Geometry: final body of the model. Coordinates: model frame, mm. Face numbers are marked on the shaded views. A direction names the side the tool comes from. Coordinates: 2 decimals unless noted, no trailing zeros. Loops run counter-clockwise (first coordinate to the right, second up) from the corner with the lowest first, then second, coordinate; pieces in that order, holes last. Notation, with made-up numbers: (-17.5, -11.5) - (-13.5, -11.5) arc R14 ccw to (-13.5, 8.5) - close; hole circle Ø8 at (5, 19.5). An arc over 180 degrees is marked (long way). Answer in a Markdown table with one row per item.
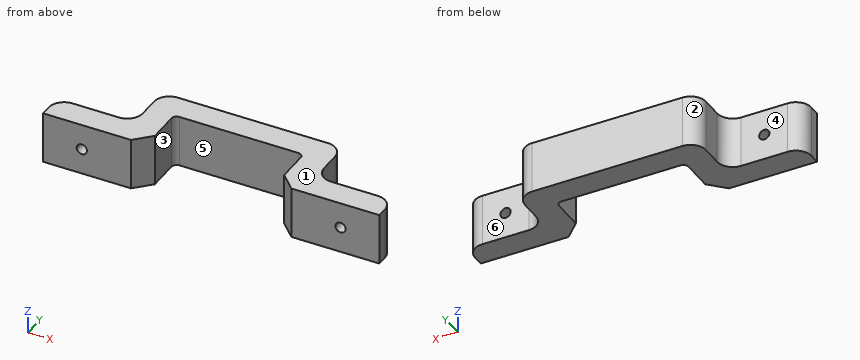
from build123d import *

# Parameters (mm, degrees)
PAD_DEPTH       = 10
FILLET_R        = 3
FILLET001_R     = 1
FILLET002_R     = 1
CHAMFER_SIZE    = 3
CHAMFER001_SIZE = 3
FILLET003_R     = 3
FILLET004_R     = 3
FILLET005_R     = 3
FILLET006_R     = 3
FILLET007_R     = 3
SKETCH001_R     = 1
POCKET_DEPTH    = 5
SKETCH002_R     = 1
POCKET001_DEPTH = 5


with BuildPart() as part:
    # Sketch → Pad (new body)
    with BuildSketch(Plane.XY):
        Polygon((0, 0), (-20, 0), (-20, 5), (-5, 5), (-5, 15), (30, 15), (30, 5), (45, 5), (45, 0), (25, 0), (25, 10), (0, 10), align=None)
    extrude(amount=PAD_DEPTH)

    # Fillet
    fillet_edges = [part.edges().sort_by_distance(p)[0] for p in [
        (-5, 15, 5),
    ]]
    fillet(fillet_edges, radius=FILLET_R)

    # Fillet001
    fillet001_edges = [part.edges().sort_by_distance(p)[0] for p in [
        (0, 10, 5),
    ]]
    fillet(fillet001_edges, radius=FILLET001_R)

    # Fillet002
    fillet002_edges = [part.edges().sort_by_distance(p)[0] for p in [
        (25, 10, 5),
    ]]
    fillet(fillet002_edges, radius=FILLET002_R)

    # Chamfer
    chamfer_edges = [part.edges().sort_by_distance(p)[0] for p in [
        (25, 0, 5),
    ]]
    chamfer(chamfer_edges, length=CHAMFER_SIZE)

    # Chamfer001
    chamfer001_edges = [part.edges().sort_by_distance(p)[0] for p in [
        (0, 0, 5),
    ]]
    chamfer(chamfer001_edges, length=CHAMFER001_SIZE)

    # Fillet003
    fillet003_edges = [part.edges().sort_by_distance(p)[0] for p in [
        (30, 15, 5),
    ]]
    fillet(fillet003_edges, radius=FILLET003_R)

    # Fillet004
    fillet004_edges = [part.edges().sort_by_distance(p)[0] for p in [
        (45, 5, 5),
    ]]
    fillet(fillet004_edges, radius=FILLET004_R)

    # Fillet005
    fillet005_edges = [part.edges().sort_by_distance(p)[0] for p in [
        (-20, 5, 5),
    ]]
    fillet(fillet005_edges, radius=FILLET005_R)

    # Fillet006
    fillet006_edges = [part.edges().sort_by_distance(p)[0] for p in [
        (30, 5, 5),
    ]]
    fillet(fillet006_edges, radius=FILLET006_R)

    # Fillet007
    fillet007_edges = [part.edges().sort_by_distance(p)[0] for p in [
        (-5, 5, 5),
    ]]
    fillet(fillet007_edges, radius=FILLET007_R)

    # Sketch001 → Pocket (cut)
    with BuildSketch(Plane(origin=(0, 5, 0), x_dir=(-1, 0, 0), z_dir=(0, 1, 0))):
        with Locations((-37.5, 5)):
            Circle(SKETCH001_R)
    extrude(amount=-POCKET_DEPTH, mode=Mode.SUBTRACT)

    # Sketch002 → Pocket001 (cut)
    with BuildSketch(Plane(origin=(0, 5, 0), x_dir=(-1, 0, 0), z_dir=(0, 1, 0))):
        with Locations((12.5, 5)):
            Circle(SKETCH002_R)
    extrude(amount=-POCKET001_DEPTH, mode=Mode.SUBTRACT)


solid = part.part
(1) Ray query, probe 1 along X at (y, z) = (9, 8.5); probe 2 along Z at (x, y) = (-12.5, 2.35); probe 3 along X at (y, z) = (11, 1.75). Return the intervals inside material, ascending.
Verdict:
| item | result |
|---|---|
| probe 1 | x = -5 to 0, 25 to 30 |
| probe 2 | z = 0 to 4, 6 to 10 |
| probe 3 | x = -5 to 30 |
(2) Cut plane A-A on z = 5. State how many separate pieces and enclosed holes the cut face has, then the cut area to 3 significant figures.
Verdict:
| item | result |
|---|---|
| separate pieces | 3 |
| enclosed holes | 0 |
| area | 393 mm² |
(3) Pull-direction query (X, two-part tool) for the marked faces 1, 2 and 3; classes: pulls with the +X half, pulls with the -X half, needs draft (parallel to the pull), parting line crosses it, or undercut.
Verdict:
| item | result |
|---|---|
| face 1 | needs draft |
| face 2 | pulls with the -X half |
| face 3 | undercut |
(4) Access query for the marked faces 4, 5 and 6. Directions: +Z, -Z, +X, -X, +Y, -Y. A direction counts if a zero-diameter tool reaches every point of the face in a straight line with its end or side. Return the directions, or none.
Verdict:
| item | result |
|---|---|
| face 4 | +Z, -Z, -X, +Y |
| face 5 | +Z, -Z, -Y |
| face 6 | +Z, -Z, +X, +Y |
(5) First-contact query: pin 1 Ø4.5 at (y, z) = (10, 7) entering from +X; pin 2 Ø1.5 at (x, z) = (24.5, 6) entering from -Y; pin 3 Ø1.2 at (x, z) = (-12.5, 5) entering from +Y; pin 4 Ø2 at (x, z) = (-11.5, 6.5) entering from +Y. Flat tips, straight axial feed; report the tip coordinate or a pass-through.
Verdict:
| item | result |
|---|---|
| pin 1 | stops at x = 30.01 |
| pin 2 | stops at y = 2.75 |
| pin 3 | passes through |
| pin 4 | stops at y = 5 |
(6) Cut plane C-C on y = 6.75. Output: boundary loops of the cut face in (x, z).
Verdict:
| item | result |
|---|---|
| outline | (-5.27, 0) - (0, 0) - (0, 10) - (-5.27, 10) - close; (25, 0) - (30.27, 0) - (30.27, 10) - (25, 10) - close |
(7) Cut plane D-D on z = 1.5. Output: boundary loops of the cut face in (x, y), then the cut area to 3 significant figures.
Verdict:
| item | result |
|---|---|
| outline | (-20, 0) - (-3, 0) - (0, 3) - (0, 9) arc R1 cw to (1, 10) - (24, 10) arc R1 cw to (25, 9) - (25, 3) - (28, 0) - (45, 0) - (45, 2) arc R3 ccw to (42, 5) - (33, 5) arc R3 cw to (30, 8) - (30, 12) arc R3 ccw to (27, 15) - (-2, 15) arc R3 ccw to (-5, 12) - (-5, 8) arc R3 cw to (-8, 5) - (-17, 5) arc R3 ccw to (-20, 2) - close |
| area | 413 mm² |
(8) Cut plane B-B on x = -12.5. Output: boundary loops of the cut face in (y, z), then the cut area to 3 significant figures.
Verdict:
| item | result |
|---|---|
| outline | (0, 0) - (5, 0) - (5, 4) - (0, 4) - close; (0, 6) - (5, 6) - (5, 10) - (0, 10) - close |
| area | 40.0 mm² |
